Verification items for this drawing (mm, ordinates from the low corner). A direction names the side the tool comes from. Coordinates: 2 decimals unless noted, no trailing zeros. Loops run counter-clockwise (first coordinate to the right, second up) from the corner with the lowest first, then second, coordinate; pieces in that order, holes last. Notation, with made-up numbers: M 46.5,-10.5 L 93.5,-10.5 A22 cw 93.5,23.5 Z; hole C 16.5,72.5 d10. An arc over 180 degrees is marked long. One line per question, with ' | ' between items. Start each with the question number.
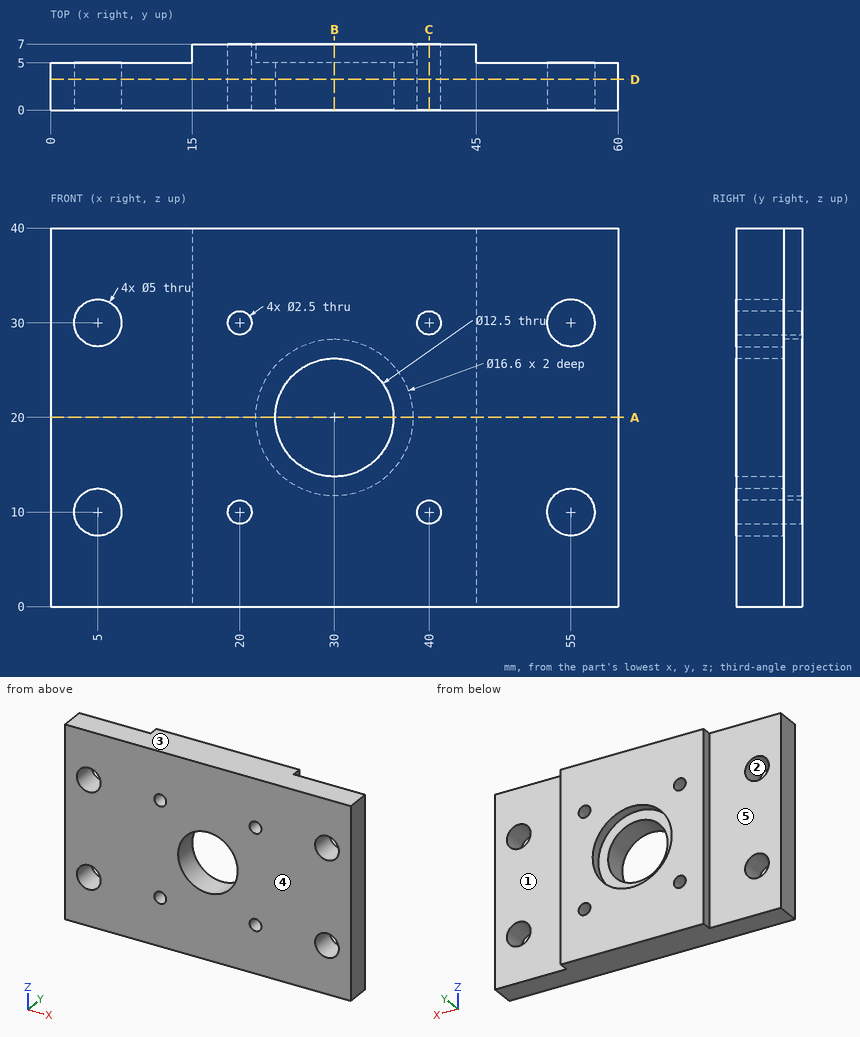
1. Sectioned sample at C-C (x = 40). Record the cut outline in (y, z).
2. Sectioned sample at A-A (z = 20). Record the cut outline in (x, y), and give its area (3 significant figures).
3. Thickness scan on line 1 (X direction, y = 2.5, z = 10); line 2 (Z direction, x = 5, y = 2.8); line 3 (Z direction, x = 7, y = 0.75). Record the ranges inside material, lowest first.
4. Depth check by flat-ended pin: pin 1 Ø3 at (x, z) = (40, 10) entering from -Y; pin 2 Ø4.5 at (x, z) = (53.5, 16.5) entering from +Y; pin 3 Ø1.6 at (y, z) = (6.5, 25.5) entering from -X; pin 4 Ø3 at (x, z) = (55, 10) entering from +Y. Enter the tip coordinate at first touch or a pass-through.
5. Sectioned sample at D-D (y = 3.25). State how many separate pieces and enclosed holes the cut face has, and give its area (3 significant figures).
6. Draft check along Z on the marked faces 1, 2 and 3. Enter one of: +Z half, -Z half, draft (parallel to the pull), parting line (faces both ways), or undercut.
7. Sectioned sample at B-B (x = 30). Record the cut outline in (y, z).
8. Tool access check on the marked faces 4 and 5. Record the directions out of +Z, -Z, +X, -X, +Y, -Y that give a thin tool (end or side, any length) a straight path to the whole face; none if there is none.
Result:
1) outline: M 0,0 L 7,0 L 7,8.75 L 0,8.75 Z; M 0,11.25 L 7,11.25 L 7,28.75 L 0,28.75 Z; M 0,31.25 L 7,31.25 L 7,40 L 0,40 Z
2) outline: M 0,0 L 23.75,0 L 23.75,5 L 21.7,5 L 21.7,7 L 15,7 L 15,5 L 0,5 Z; M 36.25,0 L 60,0 L 60,5 L 45,5 L 45,7 L 38.3,7 L 38.3,5 L 36.25,5 Z | area: 264 mm2
3) line 1: x = 0 to 2.5, 7.5 to 18.75, 21.25 to 38.75, 41.25 to 52.5, 57.5 to 60 | line 2: z = 0 to 7.5, 12.5 to 27.5, 32.5 to 40 | line 3: z = 0 to 8.5, 11.5 to 28.5, 31.5 to 40
4) pin 1: stops at y = 0 | pin 2: stops at y = 5 | pin 3: stops at x = 15 | pin 4: passes through
5) separate pieces: 1 | enclosed holes: 9 | area: 2,180 mm2
6) face 1: draft | face 2: undercut | face 3: +Z half
7) outline: M 0,0 L 7,0 L 7,11.7 L 5,11.7 L 5,13.75 L 0,13.75 Z; M 0,26.25 L 5,26.25 L 5,28.3 L 7,28.3 L 7,40 L 0,40 Z
8) face 4: +Z, -Z, +X, -X, -Y | face 5: +Z, -Z, -X, +Y
